Geometry: final body of the model. Coordinates: model frame, mm. Face numbers are marked on the shaded views. A direction names the side the tool comes from. Give positions to 0.01 mm unless a question says otherwise; leave off trailing zeros. Write each loop counter-clockwise with the first axis right and the second up, starting at its lowest first coordinate (ties: lowest second). Pieces come first, ordered by that corner, then holes. Notation, with made-up numbers: M 25,-31.75 L 46,-31.75 A32 ccw 46,-2.75 Z; hole C 9.25,59 d2. An arc over 180 degrees is marked long. Use one line per item in the form item = value. Start each with the question number.
Item 1: Contact query for flat-ended pins moving along their axis: P1, Ø2, axis at y = -8, z = -6.5, coming from the -X side; P2, Ø2, axis at x = 8, z = 9, coming from the +Y side; P3, Ø3.5, axis at y = -32, z = -12, coming from the -X side. Output: stop coordinate, or through.
Item 2: Section query D-D on x = 6. Return loops of the section in (y, z), then the cut area to 3 significant figures.
Item 3: Pull-direction query (X, two-part tool) for the marked faces 3, 4, 5 and 6; classes: released by +X, released by -X, zero draft, split by the parting line, or undercut.
Item 4: Section query A-A on z = -9. Return loops of the section in (x, y).
Item 5: Material intervals for line 1 along Z through (x, y) = (5.75, -34.75); line 2 along Z through (x, y) = (1.65, -34.75); line 3 along X through (y, z) = (-20.5, -16), sorted ascending. Write a range as from..to.
Item 6: Access query for the marked faces 1 and 2. Directions: +Z, -Z, +X, -X, +Y, -Y. A direction counts if a zero-diameter tool reaches every point of the face in a straight line with its end or side. Return the directions, or none.
Item 7: Section query C-C on y = -4. Return loops of the section in (x, z).
Item 8: Section query B-B on y = -34.75. Return loops of the section in (x, z).
from build123d import *

# Parameters (mm, degrees)
RESSALTO_EXTRUS_O1_DEPTH                             = 19
FILETE1_R                                            = 1.5
RESSALTO_EXTRUS_O2_DEPTH                             = 2.5
REBAIXO_PARA_PARAFUSO_ALLEN_SEXTAVADO_DE_D           = 5.5
REBAIXO_PARA_PARAFUSO_ALLEN_SEXTAVADO_DE_CBORE_D     = 11.5
REBAIXO_PARA_PARAFUSO_ALLEN_SEXTAVADO_DE_CBORE_DEPTH = 3


with BuildPart() as part:
    # Esboço1 → Ressalto-extrusão1 (new, symmetric)
    with BuildSketch(Plane.XY):
        with BuildLine():
            Line((0, 0), (0, -30))
            ThreePointArc((0, -30), (3.840309651, -42.417932709), (14.020349891, -50.5))
            Line((14.020349891, -50.5), (15.7, -48.014285714))
            ThreePointArc((15.7, -48.014285714), (8.658133916, -34.757142857), (15.7, -21.5))
            Line((15.7, -21.5), (14.5, -9))
            Line((14.5, -9), (9.5, -9))
            Line((9.5, -9), (9.5, -21.5))
            Line((9.5, -21.5), (5, -21.5))
            Line((5, -21.5), (5, 0))
            Line((5, 0), (0, 0))
        make_face()
    extrude(amount=RESSALTO_EXTRUS_O1_DEPTH, both=True)

    # Filete1
    filete1_edges = [part.edges().sort_by_distance(p)[0] for p in [
        (5, 0, 0),
        (9.5, -9, 0),
        (14.5, -9, 0),
        (15.7, -21.5, 0),
        (15.7, -48.014285714, 0),
        (14.020349891, -50.5, 0),
        (0, 0, 0),
    ]]
    fillet(filete1_edges, radius=FILETE1_R)

    # Esboço3 → Ressalto-extrusão2 (add, symmetric)
    with BuildSketch(Plane.XY):
        with BuildLine():
            Line((0, -1.5), (-5, -6.5))
            Line((-5, -6.5), (-5, -24.5))
            ThreePointArc((-5, -24.5), (-0.096122461, -40.062531476), (12.8437502, -50.002355236))
            ThreePointArc((12.8437502, -50.002355236), (3.487375513, -41.885454705), (0, -30))
            Line((0, -30), (0, -1.5))
        make_face()
    extrude(amount=RESSALTO_EXTRUS_O2_DEPTH, both=True)

    # Rebaixo para parafuso Allen sextavado de M51 (through all)
    with Locations(Plane.ZY):
        with Locations((-9.5, -34.75), (9.5, -34.75)):
            CounterBoreHole(REBAIXO_PARA_PARAFUSO_ALLEN_SEXTAVADO_DE_D / 2, REBAIXO_PARA_PARAFUSO_ALLEN_SEXTAVADO_DE_CBORE_D / 2, REBAIXO_PARA_PARAFUSO_ALLEN_SEXTAVADO_DE_CBORE_DEPTH)


solid = part.part
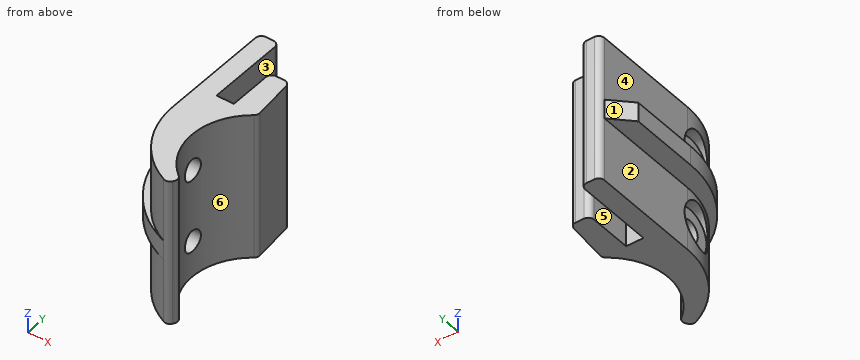
Answer sheet:
q1.P1 = 0
q1.P2 = -21.5
q1.P3 = 3
q2.outline = M -46.32,-2.5 L -45.1,-2.5 L -45.1,-19 L -21.5,-19 L -21.5,19 L -45.1,19 L -45.1,2.5 L -46.32,2.5 Z; hole C -34.75,-9.5 d5.5; hole C -34.75,9.5 d5.5
q2.area = 855 mm2
q3.face_3 = undercut
q3.face_4 = released by -X
q3.face_5 = undercut
q3.face_6 = released by +X
q4.outline = M 0,-29.02 L 3,-29.02 L 3,-32.05 L 8.89,-32.05 A16 cw 15.03,-21.98 A1.5 ccw 15.62,-20.64 L 14.63,-10.36 A1.5 ccw 13.14,-9 L 11,-9 A1.5 ccw 9.5,-10.5 L 9.5,-21.5 L 5,-21.5 L 5,-1.5 A1.5 ccw 3.5,0 L 1.5,0 A1.5 ccw 0,-1.5 Z; M 2.66,-40.48 A22 ccw 12.84,-50 A1.5 ccw 14.71,-49.48 L 14.9,-49.2 A1.5 ccw 14.6,-47.2 A16 cw 8.89,-37.45 L 3,-37.45 L 3,-40.48 Z
q5.line_1 = -19..-12.25, -6.75..6.75, 12.25..19
q5.line_2 = -19..-15.25, -3.75..3.75, 15.25..19
q5.line_3 = 0..5, 9.5..15.6
q6.face_1 = +Z, -Z, -X, +Y
q6.face_2 = -Z, -X, +Y, -Y
q7.outline = M -2.5,-2.5 L 0,-2.5 L 0,-19 L 5,-19 L 5,19 L 0,19 L 0,2.5 L -2.5,2.5 Z
q8.outline = M -2.99,-2.5 L 0.52,-2.5 L 0.52,-3.75 L 3,-3.75 L 3,-6.75 L 8.66,-6.75 L 8.66,6.75 L 3,6.75 L 3,3.75 L 0.52,3.75 L 0.52,2.5 L -2.99,2.5 Z; M 0.52,-19 L 8.66,-19 L 8.66,-12.25 L 3,-12.25 L 3,-15.25 L 0.52,-15.25 Z; M 0.52,15.25 L 3,15.25 L 3,12.25 L 8.66,12.25 L 8.66,19 L 0.52,19 Z
